Answer from the drawing. Dimensions are ordinates in mm from the lowest x, y and z of the part. Round coordinates to 2 decimals unless told otherwise and drop trailing zeros. Loops run counter-clockwise (first coordinate to the right, second up) from the corner with the lowest first, then second, coordinate; pieces in that order, holes last. Notation, with made-up numbers: (68.25, -17) - (114.25, -17) arc R23 cw to (114.25, 19) - close; hole circle Ø4 at (63.25, 47). An arc over 180 degrees is marked (long way). Return JSON: item names as keys, results as strings.
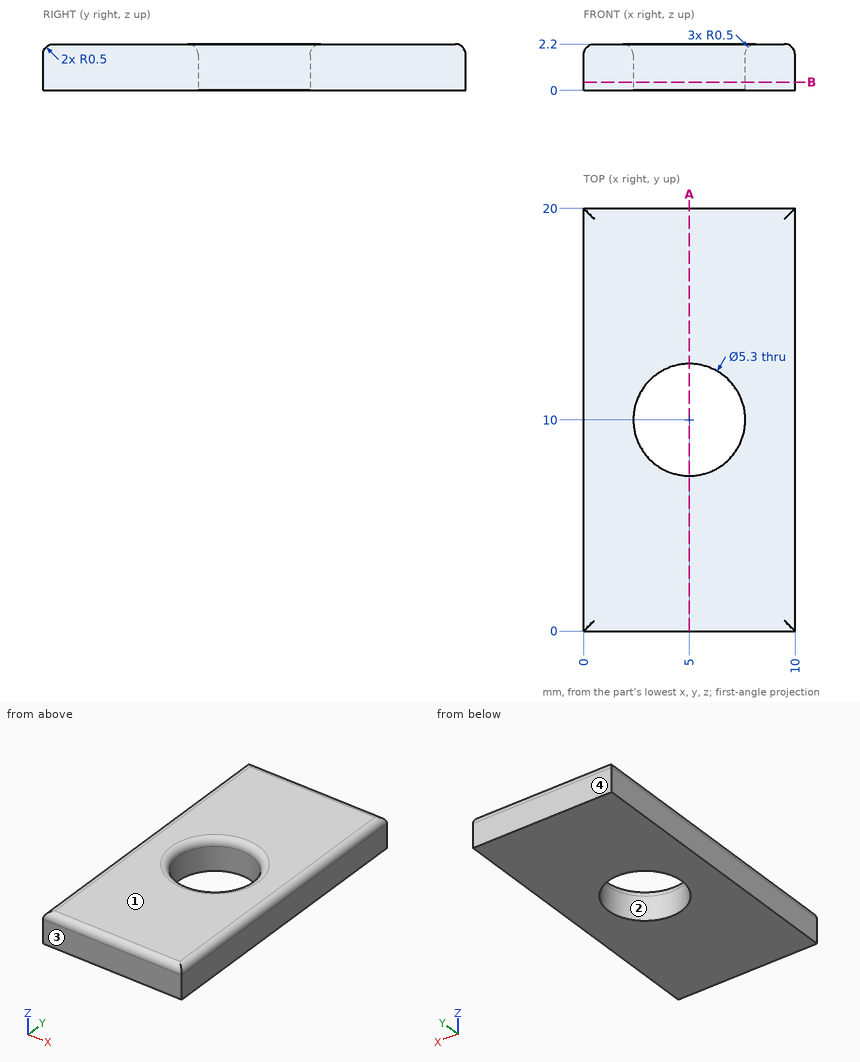
1) Section A-A (x = 5) is taken. Give the vertices of the cut face in (y, z), and give its area (3 significant figures).
Verdict:
{"outline": "(0, 0) - (7.35, 0) - (7.35, 1.7) arc R0.5 ccw to (6.85, 2.2) - (0.5, 2.2) arc R0.5 ccw to (0, 1.7) - close; (12.65, 0) - (20, 0) - (20, 1.7) arc R0.5 ccw to (19.5, 2.2) - (13.15, 2.2) arc R0.5 ccw to (12.65, 1.7) - close", "area": "32.1 mm2"}
2) Section B-B (z = 0.4) is taken. Give the vertices of the cut face in (x, y).
Verdict:
{"outline": "(0, 0) - (10, 0) - (10, 20) - (0, 20) - close; hole circle Ø5.3 at (5, 10)"}
3) Determine the mould class of the marked faces 1, 2, 3 and 4 for opening direction Y: pulls with the +Y half, pulls with the -Y half, needs draft (parallel to the pull), parting line crosses it, or undercut.
Verdict:
{"face 1": "needs draft", "face 2": "undercut", "face 3": "pulls with the -Y half", "face 4": "pulls with the +Y half"}
4) Find the intervals of material crossed by L1, parallel to Y at x = 6, z = 0.55; L2, parallel to Y at x = 5.75, z = 1.8; L3, parallel to X at y = 11.5, z = 0.6, in increasing order.
Verdict:
{"L1": "y = 0 to 7.55, 12.45 to 20", "L2": "y = 0.01 to 7.45, 12.55 to 19.99", "L3": "x = 0 to 2.82, 7.18 to 10"}
